Part model, mm, in its own coordinate system. Face numbers are marked on the shaded views. A direction names the side the tool comes from. Coordinates: 2 decimals unless noted, no trailing zeros. Loops run counter-clockwise (first coordinate to the right, second up) from the corner with the lowest first, then second, coordinate; pieces in that order, holes last. Notation, with made-up numbers: M -40,62.5 L 14,62.5 A36 cw 14,98.5 Z; hole C -19.75,55 d7. An arc over 180 degrees is marked long. Use a Markdown table: item, result. Add a question column.
1) Band-saw the part on D-D (y = -70.5). List the corners of the cut face in (x, z), plus the area to 3 significant figures.
2) Band-saw the part on C-C (z = -34). List the corners of the cut face in (x, y).
3) Pull direction X, two halves, no side cores. Call the marked faces 3, 4 and 5: released by +X, released by -X, zero draft, split by the parting line, or undercut.
4) Pin check, flat tips, straight feed: pin 1 Ø4 at (x, y) = (48, -82) entering from +Z; pin 2 Ø2 at (x, y) = (28, -28.5) entering from +Z; pin 3 Ø8 at (x, y) = (-54.5, -82.5) entering from +Z. Stop position of each tip, or through.
5) Wall check: probe 1 along X at (y, z) = (-50.5, -14); probe 2 along Y at (x, z) = (-16.5, -23); probe 3 along Y at (x, z) = (56, 11.5). Give the ranges that are in metal, low to high. Write a range as from..to.
6) Band-saw the part on B-B (z = -59). List the corners of the cut face in (x, y).
7) Tool access for the marked faces 1 and 2: list every direction of +Z, -Z, +X, -X, +Y, -Y with a clear straight run to the whole face (end or side of a thin tool).
8) Band-saw the part on A-A (y = 31). List the corners of the cut face in (x, z).
from build123d import *

# Parameters (mm, degrees)
F1_DEPTH = 89.1325119883
F3_DEPTH = 77.1384909749
F4_DEPTH = 218.7686692923
F5_T     = -2.54
F6_R     = 15.5818396181
F7_R     = 3.0969406223


with BuildPart() as f1:
    # F0 (on Front) → F1 (new body)
    with BuildSketch(Plane.XZ):
        Polygon((-77.014118433, 0), (-77.014118433, -76.4366090298), (76.849937439, -76.4366090298), (76.849937439, 0), (62.097877264, 8.7319239974), (41.6193008423, 45.3698374331), (-39.5245552063, 45.4712845385), (-59.4715923071, 8.7319239974), align=None)
    extrude(amount=-F1_DEPTH)

    # F2 (on Right) → F3 (join, symmetric)
    with BuildSketch(Plane.YZ):
        Polygon((0, -76.6211944324), (0, 46.0868030787), (-24.9364376068, 0), (-125.2473463191, -10.5374917338), (-125.8752644062, -75.4026770592), align=None)
    extrude(amount=F3_DEPTH, both=True)

    # F4 (cut): a face of the model
    f4_faces = [f1.faces().sort_by_distance(p)[0] for p in [
        (76.9413650258, 0, -15.2671956769),
    ]]
    extrude(f4_faces, amount=-F4_DEPTH, mode=Mode.SUBTRACT)

    # F5
    f5_openings = [f1.faces().sort_by_distance(p)[0] for p in [
        (-0.08209, -72.471652, -75.919643),
        (-0.08209, 35.032237, -76.436609),
    ]]
    offset(amount=F5_T, openings=f5_openings, kind=Kind.INTERSECTION)

    # F6
    f6_edges = [f1.edges().sort_by_distance(p)[0] for p in [
        (-0.08209, -24.936438, 0),
    ]]
    fillet(f6_edges, radius=F6_R)

    # F7
    f7_edges = [f1.edges().sort_by_distance(p)[0] for p in [
        (-49.498074, -10.272425, 27.101604),
        (51.858589, -10.29987, 27.050881),
        (1.047373, -0.360487, 45.420561),
        (41.619301, 44.37229, 45.369837),
        (-39.524555, 44.399735, 45.471285),
    ]]
    fillet(f7_edges, radius=F7_R)


solid = f1.part
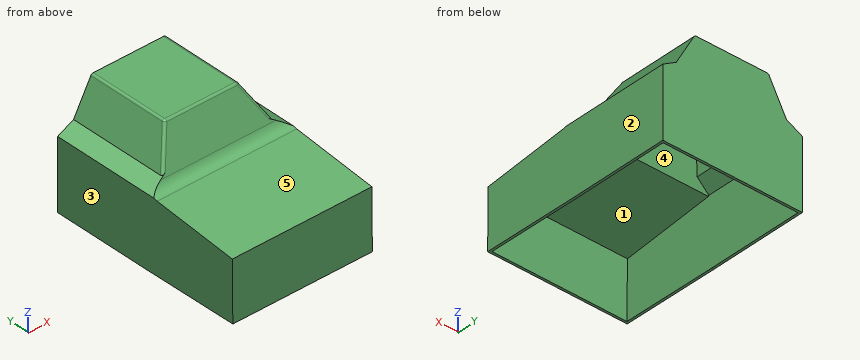
Entries:
| question | item | result |
|---|---|---|
| 1 | outline | M -77.01,-75.94 L -74.47,-75.94 L -74.47,-7.34 L 74.31,-7.34 L 74.31,-75.94 L 76.85,-75.94 L 76.85,-4.79 L -77.01,-4.79 Z |
| 1 | area | 741 mm2 |
| 2 | outline | M -77.01,-125.47 L 76.85,-125.47 L 76.85,89.13 L -77.01,89.13 Z; hole M -74.47,-122.93 L 74.31,-122.93 L 74.31,86.59 L -74.47,86.59 Z |
| 3 | face 3 | released by -X |
| 3 | face 4 | undercut |
| 3 | face 5 | zero draft |
| 4 | pin 1 | z = -5.78 |
| 4 | pin 2 | z = 0.84 |
| 4 | pin 3 | z = -5.63 |
| 5 | probe 1 | -77.01..-74.47, 74.31..76.85 |
| 5 | probe 2 | -125.37..-122.83, 86.59..89.13 |
| 5 | probe 3 | -18.71..-15.83, 86.59..89.13 |
| 6 | outline | M -77.01,-125.72 L 76.85,-125.72 L 76.85,89.13 L -77.01,89.13 Z; hole M -74.47,-123.18 L 74.31,-123.18 L 74.31,86.59 L -74.47,86.59 Z |
| 7 | face 1 | -Z |
| 7 | face 2 | +Z, -Z, +X, +Y, -Y |
| 8 | outline | M -77.01,-76.44 L -74.47,-76.44 L -74.47,-1.57 L -57.62,6.82 L -38.01,42.93 L 40.13,42.83 L 60.21,6.89 L 74.31,-1.45 L 74.31,-76.44 L 76.85,-76.44 L 76.85,0 L 62.1,8.73 L 42.5,43.79 A3.1 ccw 39.81,45.37 L -37.68,45.47 A3.1 ccw -40.4,43.85 L -59.47,8.73 L -77.01,0 Z |
